CAD build for the part. Positions are in the model's coordinates, mm. A direction names the side the tool comes from. Coordinates: 2 decimals unless noted, no trailing zeros. Loops run counter-clockwise (first coordinate to the right, second up) from the corner with the lowest first, then second, coordinate; pieces in that order, holes last. Notation, with made-up numbers: (41.5, -1.75) -> (47.5, -1.75) arc R22 ccw to (47.5, 6.25) -> close; hole circle Ø7 at (-26, 88). An arc over 180 degrees is marked (long way). Return JSON: item names as keys, results as strings. Group by question number.
(1) Mould opens along Z. For faces 1 (the face through (-23.448, 0.187, -1.103)), 2 (the face through (-12.87, -3.02, -2.5)), 3 (the face through (-13.1, -2.4, -4)) say: pulls with the +Z half, pulls with the -Z half, needs draft (parallel to the pull), parting line crosses it, or undercut.
(2) Flat gauge pins, fed straight in: pin 1 Ø1.5 at (y, z) = (1.5, -3.5) entering from -X; pin 2 Ø4 at (x, y) = (-4, -6.5) entering from -Z; pin 3 Ø3 at (y, z) = (-2.5, -2) entering from -X. Where does each tip first touch, or does it go through?
(3) Probe L1, parallel to Y at x = 14.5, z = -3.9; L2, parallel to X at y = 0, z = -4.05; L3, parallel to Z at x = 3, y = -1.25. List the from-to ranges inside material, lowest first.
(4) Saw through at A-A on z = -1.85. Write the cut outline in (x, y) (3 decimals), then the cut area to 3 significant figures.
(5) Tool access for faces 4 (the face through (-15.9, 2.4, -2.5)), 5 (the face through (-14.5, 3, -3)), 6 (the face through (17.98, 1.09, -0.86)): list every direction of +Z, -Z, +X, -X, +Y, -Y with a clear straight run to the whole face (end or side of a thin tool).
```python
from build123d import *

# Parameters (mm, degrees)
F1_DEPTH         = 1.6
F4_DEPTH         = 1.3
F5_SIZE2         = 1.3
F5_SIZE          = 0.9
F5_2_SIZE2       = 1.29999
F5_2_SIZE        = 0.89999
F6_R             = 4.5
F6_R_2           = 3.26
F7_DEPTH         = 3
F8_DEPTH         = 2.901
F9_R             = 3.645
F9_R_2           = 3.26
F10_DEPTH        = 5
F11_W            = 0.8
F11_H            = 1.2
F13_ANGLE_BACK   = 30
F13_ANGLE        = 60
F13_COPIES_COUNT = 3
F14_ANGLE_BACK   = 15
F14_ANGLE        = 30
F14_COPIES_COUNT = 3
F15_R            = 0.3


# Not quite as in the source:
# - a fillet or chamfer is up to 0.001 mm smaller than in the source, because OpenCascade refuses the exact size
# - after a boolean that leaves OpenCascade's solid faulty, fix() repairs it
# - a pattern or mirror of a feature is missing from the dataset's text; its kind, count and spacing are read off the source's solid


with BuildPart() as f1:
    # F0 (on Top) → F1 (new body)
    with BuildSketch(Plane.XY):
        with BuildLine():
            Line((14.95, 5.9), (-14.95, 5.9))
            ThreePointArc((-14.95, 5.9), (-20.85, 0), (-14.95, -5.9))
            Line((-14.95, -5.9), (14.95, -5.9))
            ThreePointArc((14.95, -5.9), (20.85, 0), (14.95, 5.9))
        make_face()
    extrude(amount=F1_DEPTH)

    # F3 (on offset) → F4 (join)
    with BuildSketch(Plane.XY.offset(-1.3)):
        with BuildLine():
            Line((14.95, 8.5), (-14.95, 8.5))
            ThreePointArc((-14.95, 8.5), (-23.45, 0), (-14.95, -8.5))
            Line((-14.95, -8.5), (14.95, -8.5))
            ThreePointArc((14.95, -8.5), (23.45, 0), (14.95, 8.5))
        make_face()
    extrude(amount=F4_DEPTH)

    # F5
    f5_edges = [f1.edges().sort_by_distance(p)[0] for p in [
        (0, 8.5, 0),
    ]]
    f5_side = f1.faces().sort_by_distance((0, 8.5, -0.65))[0]
    chamfer(f5_edges, length=F5_SIZE, length2=F5_SIZE2, reference=f5_side)

    # F5#2 (size 0.9 and 1.3 in the source; OpenCascade refuses exactly that, so slightly less here)
    f5_2_edges = [f1.edges().sort_by_distance(p)[0] for p in [
        (0, -5.9, 0),
    ]]
    f5_2_side = f1.faces().sort_by_distance((0, -5.9, 0.8))[0]
    chamfer(f5_2_edges, length=F5_2_SIZE, length2=F5_2_SIZE2, reference=f5_2_side)

    # F6 (on face) → F7 (join)
    with BuildSketch(Plane(origin=(0, 0, -1.3), x_dir=(1, 0, 0), z_dir=(0, 0, -1))):
        with Locations((14.5, 0)):
            Circle(F6_R)
        with Locations((14.5, 0)):
            Circle(F6_R_2, mode=Mode.SUBTRACT)
    extrude(amount=F7_DEPTH)

    # F8 (cut, through all): a face of the model
    f8_faces = [f1.faces().sort_by_distance(p)[0] for p in [
        (14.5, 0, -1.3),
    ]]
    extrude(f8_faces, amount=-F8_DEPTH, mode=Mode.SUBTRACT)

    # F9 (on face) → F10 (cut)
    with BuildSketch(Plane.XY.offset(1.6)):
        with Locations((14.5, 0)):
            Circle(F9_R)
        with Locations((14.5, 0)):
            Circle(F9_R_2, mode=Mode.SUBTRACT)
    extrude(amount=-F10_DEPTH, mode=Mode.SUBTRACT)

    # F11 (on Front) → F12 (revolve)
    with BuildSketch(Plane.XZ):
        with Locations((-17.35, -1.9)):
            Rectangle(F11_W, F11_H)
    revolve(axis=Axis((-14.5, 0, 1.6), (0, 0, 1)))

    # F11 (on Front) → F13 (revolve)
    with BuildSketch(Plane.XZ, mode=Mode.PRIVATE) as f13_sk:
        Polygon((-16.95, -4), (-16.95, -2.5), (-17.75, -2.5), (-18.55, -2.5), (-17.75, -4), align=None)
    f13 = revolve(f13_sk.sketch.rotate(Axis((-14.5, 0, 1.6), (0, 0, 1)), -F13_ANGLE_BACK), axis=Axis((-14.5, 0, 1.6), (0, 0, 1)), revolution_arc=F13_ANGLE)

    # F13_copies: F13 ×3 about axis
    f13_copies_axis = Axis((-14.5, 0, 0), (0, 0, 1))
    for i in range(1, F13_COPIES_COUNT):
        add(f13.rotate(f13_copies_axis, i * 360 / F13_COPIES_COUNT))

    # F11 (on Front) → F14 (revolve)
    with BuildSketch(Plane.XZ, mode=Mode.PRIVATE) as f14_sk:
        Polygon((-16.15, -1.3), (-16.95, -1.3), (-16.95, -2.5), align=None)
    f14 = revolve(f14_sk.sketch.rotate(Axis((-14.5, 0, 1.6), (0, 0, 1)), -F14_ANGLE_BACK), axis=Axis((-14.5, 0, 1.6), (0, 0, 1)), revolution_arc=F14_ANGLE)

    # F14_copies: F14 ×3 about axis
    f14_copies_axis = Axis((-14.5, 0, 0), (0, 0, 1))
    for i in range(1, F14_COPIES_COUNT):
        add(f14.rotate(f14_copies_axis, i * 360 / F14_COPIES_COUNT))

    add(f1.part.fix(), mode=Mode.REPLACE)

    # F15
    f15_edges = [f1.edges().sort_by_distance(p)[0] for p in [
        (10, 0, -4.3),
    ]]
    fillet(f15_edges, radius=F15_R)


solid = f1.part
```
Geometry results:
{
 "1": {"face 1": "needs draft", "face 2": "undercut", "face 3": "pulls with the -Z half"},
 "2": {"pin 1": "x = -18.2", "pin 2": "z = -1.3", "pin 3": "x = -23.37"},
 "3": {"L1": "-4.5 to -3.26, 3.26 to 4.5", "L2": "10 to 11.24, 17.76 to 19", "L3": "-1.3 to 1.6"},
 "4": {"outline": "circle Ø6.5 at (-14.5, 0); circle Ø9 at (14.5, 0); hole (-16.867, -0.634) arc R2.45 ccw to (-13.866, -2.367) -> (-13.978, -1.948) arc R2.017 ccw to (-13.074, -1.426) -> (-12.768, -1.732) arc R2.45 ccw to (-12.768, 1.732) -> (-13.074, 1.426) arc R2.017 ccw to (-13.978, 1.948) -> (-13.866, 2.367) arc R2.45 ccw to (-16.867, 0.634) -> (-16.448, 0.522) arc R2.017 ccw to (-16.448, -0.522) -> close; hole circle Ø7.29 at (14.5, 0)", "area": "37.7 mm²"},
 "5": {"face 4": "-Z, +Y", "face 5": "-Z, -X, +Y, -Y", "face 6": "+Z"}
}
